Geometry check sheet. Reference: the model listing, model coordinates, mm. Face numbers are marked on the shaded views. Coordinates: 2 decimals unless noted, no trailing zeros. Write each loop counter-clockwise with the first axis right and the second up, starting at its lowest first coordinate (ties: lowest second). Pieces come first, ordered by that corner, then holes. Notation, with made-up numbers: (-23, 7) -> (19, 7) arc R29 ccw to (19, 45) -> close; hole circle Ø9 at (-26.5, 40.25). An arc over 180 degrees is marked (long way). Answer in a Markdown table with one row per item. Add a question column.
1. Scan lines: L1, parallel to Y at x = 0, z = 20.5; L2, parallel to Z at x = 18, y = 2.5; L3, parallel to Z at x = -20.5, y = -11.5. Record each from-to range of solid material in increasing order. Write a range as from..to.
2. Cross-section at C-C on z = 23. Record the cut outline in (x, y), and give its area (3 significant figures).
3. Mould release check, pull along Z, two halves, no side actions. Record for the marked faces 1, 2, 3 and 4: pulls with the +Z half, pulls with the -Z half, needs draft (parallel to the pull), parting line crosses it, or undercut.
4. Depth check by flat-ended pin: P1, Ø8, axis at x = 15, z = 15, coming from the +Y side; P2, Ø5, axis at y = 13, z = 14.5, coming from the +X side; P3, Ø8, axis at y = -5, z = 16, coming from the -X side. Enter the tip coordinate at first touch or a pass-through.
5. Cross-section at A-A on y = 0. Record the cut outline in (x, z).
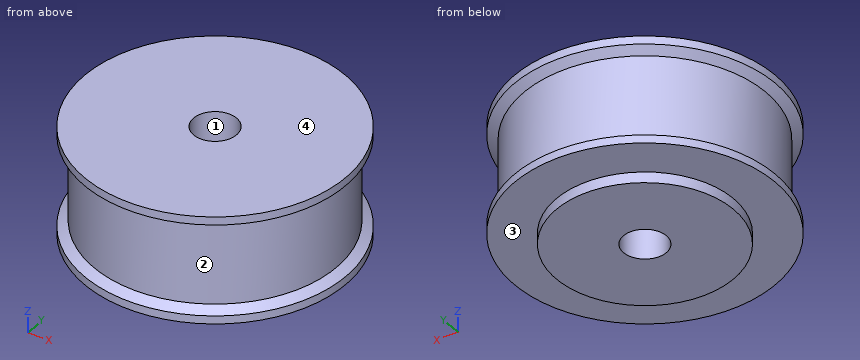
```python
from build123d import *

# Parameters (mm, degrees)
SKICA2_W                 = 8
SKICA2_H                 = 33
ODEBRAT_VYSUNUT_M1_DEPTH = 35


with BuildPart() as part:
    # Skica1 → Rotovat1 (revolve)
    with BuildSketch(Plane(origin=(0, 0, 0), x_dir=(0, 0, -1), z_dir=(1, 0, 0)), mode=Mode.PRIVATE) as rotovat1_sk:
        Polygon((0, 4), (0, 16.5), (-10, 16.5), (-10, 24.28), (-11.5, 24.28), (-12.5, 22.54), (-27.5, 22.54), (-28.5, 24.28), (-30, 24.28), (-30, 4), align=None)
    revolve(rotovat1_sk.sketch.rotate(Axis((0, 0, 0), (0, 0, 1)), 90), axis=Axis((0, 0, 0), (0, 0, 1)))

    # Skica2 → Odebrat vysunutím1 (cut, symmetric)
    with BuildSketch(Plane(origin=(0, 0, 0), x_dir=(0, 0, -1), z_dir=(1, 0, 0))):
        with Locations((-4, 0)):
            Rectangle(SKICA2_W, SKICA2_H)
    extrude(amount=ODEBRAT_VYSUNUT_M1_DEPTH, both=True, mode=Mode.SUBTRACT)


solid = part.part
```
Results found:
| question | item | result |
|---|---|---|
| 1 | L1 | y = -22.54..-4, 4..22.54 |
| 1 | L2 | z = 10..30 |
| 1 | L3 | z = 10..11.95, 28.05..30 |
| 2 | outline | circle Ø45.08 at (0, 0); hole circle Ø8 at (0, 0) |
| 2 | area | 1,550 mm^2 |
| 3 | face 1 | needs draft |
| 3 | face 2 | undercut |
| 3 | face 3 | pulls with the -Z half |
| 3 | face 4 | pulls with the +Z half |
| 4 | P1 | stops at y = 20.47 |
| 4 | P2 | stops at x = 19.94 |
| 4 | P3 | stops at x = -22.92 |
| 5 | outline | (-24.28, 10) -> (-16.5, 10) -> (-16.5, 8) -> (-4, 8) -> (-4, 30) -> (-24.28, 30) -> (-24.28, 28.5) -> (-22.54, 27.5) -> (-22.54, 12.5) -> (-24.28, 11.5) -> close; (4, 8) -> (16.5, 8) -> (16.5, 10) -> (24.28, 10) -> (24.28, 11.5) -> (22.54, 12.5) -> (22.54, 27.5) -> (24.28, 28.5) -> (24.28, 30) -> (4, 30) -> close |
